Input: part model. Units: mm. Frame: model coordinates. A direction names the side the tool comes from. Coordinates: 2 decimals unless noted, no trailing zeros. Order: outer loops, then holes, each group sorted by start corner. A loop starts at its lowest first (then second) coordinate and runs counter-clockwise, first axis right, second up. Notation, with made-up numbers: (56, 32) - (73, 32) arc R23 cw to (73, 59) - close; hole circle Ø5 at (-23, -36.5). An arc over 180 degrees is marked (long way). One line per question, with ' | ' between items. Start each with the question number.
```python
from build123d import *

# Parameters (mm, degrees)
F0_W     = 5.5
F0_H     = 22
F2_R     = 5.2
F3_DEPTH = 3
F4_R     = 2.6
F5_DEPTH = 25


with BuildPart() as f1:
    # F0 (on Front) → F1 (revolve)
    with BuildSketch(Plane.XZ):
        with Locations((5.199999, 31.5)):
            Rectangle(F0_W, F0_H)
    revolve(axis=Axis((-4.686111, 0, 0), (-1, 0, 0)))

    # F2 (on face) → F3 (cut)
    with BuildSketch(Plane.YZ.offset(7.949999)):
        with Locations((0, 35)):
            Circle(F2_R)
        with Locations((0, -35)):
            Circle(F2_R)
    extrude(amount=-F3_DEPTH, mode=Mode.SUBTRACT)

    # F4 (on face) → F5 (cut)
    with BuildSketch(Plane.YZ.offset(4.949999)):
        with Locations((0, 35)):
            Circle(F4_R)
        with Locations((0, -35)):
            Circle(F4_R)
    extrude(amount=-F5_DEPTH, mode=Mode.SUBTRACT)


solid = f1.part
```
(1) Reachability of faces 1 (the face through (4.95, 2, 33)), 2 (the face through (7.95, -18.3, 10)) from +Z, -Z, +X, -X, +Y, -Y: full face, straight path, thin tool, end or side. Return the list, or none.
(2) Draft query along Z for faces 3 (the face through (4.95, 2, -37)), 4 (the face through (5.238, -25.861, -33.727)), 5 (the face through (2.45, -18.3, 10)). Return one class per face: +Z half, -Z half, draft (parallel to the pull), parting line (faces both ways), or undercut.
(3) Section D-D (x = 5.9). Output: boundary loops of the cut face in (y, z).
(4) Material intervals for line 1 along Y through (x, z) = (5.85, 0); line 2 along Z through (x, y) = (5.4, -7); line 3 along Y through (x, z) = (3.9, 9), sorted ascending. Write a range as from..to.
(5) Section C-C (y = -16.5). Output: boundary loops of the cut face in (x, z), then the cut area to 3 significant figures.
(6) Pin query (flat end, axial travel): pin 1 (8.5 mm diameter, centred on y = 0.5, z = -34.5, fed in from +X); pin 2 (2 mm diameter, centred on x = 6.5, z = -12.5, fed in from -Y). Return the tip coordinate at first contact, or that it passes through.
(7) Section B-B (y = 0). Output: boundary loops of the cut face in (x, z).
(8) Section A-A (z = 0). Output: boundary loops of the cut face in (x, y), then the cut area to 3 significant figures.
Worked answers:
1) face 1: +X | face 2: +Z, -Z, +X, +Y, -Y
2) face 3: undercut | face 4: parting line | face 5: draft
3) outline: circle Ø85 at (0, 0); hole circle Ø41 at (0, 0); hole circle Ø10.4 at (0, -35); hole circle Ø10.4 at (0, 35)
4) line 1: y = -42.5..-20.5, 20.5..42.5 | line 2: z = -41.92..-19.27, 19.27..41.92 | line 3: y = -41.54..-18.42, 18.42..41.54
5) outline: (2.45, -39.17) - (7.95, -39.17) - (7.95, -12.17) - (2.45, -12.17) - close; (2.45, 12.17) - (7.95, 12.17) - (7.95, 39.17) - (2.45, 39.17) - close | area: 297 mm²
6) pin 1: stops at x = 4.95 | pin 2: stops at y = -40.91
7) outline: (2.45, -42.5) - (7.95, -42.5) - (7.95, -40.2) - (4.95, -40.2) - (4.95, -37.6) - (2.45, -37.6) - close; (2.45, -32.4) - (4.95, -32.4) - (4.95, -29.8) - (7.95, -29.8) - (7.95, -20.5) - (2.45, -20.5) - close; (2.45, 20.5) - (7.95, 20.5) - (7.95, 29.8) - (4.95, 29.8) - (4.95, 32.4) - (2.45, 32.4) - close; (2.45, 37.6) - (4.95, 37.6) - (4.95, 40.2) - (7.95, 40.2) - (7.95, 42.5) - (2.45, 42.5) - close
8) outline: (2.45, -42.5) - (7.95, -42.5) - (7.95, -20.5) - (2.45, -20.5) - close; (2.45, 20.5) - (7.95, 20.5) - (7.95, 42.5) - (2.45, 42.5) - close | area: 242 mm²
